Read the model definition and answer for the solid it produces. Units are mm, in the model's axes. Face numbers are marked on the shaded views. Round coordinates to 2 decimals unless told otherwise and drop trailing zeros. Order: outer loops, then holes, each group sorted by start corner. A loop starts at its lowest first (then second) coordinate and runs counter-clockwise, first axis right, second up. Notation, with made-up numbers: (31, 79) -> (52, 79) arc R35 ccw to (52, 113) -> close; hole circle Ø2 at (-39, 24). An arc over 180 degrees is marked (long way). Answer as a JSON object with one key per item and string values. Group by question number.
Item 1: Consider probe 1 along Z at (x, y) = (69, 1.2); probe 2 along X at (y, z) = (1.9, 99); probe 3 along X at (y, z) = (0.6, 98). Determine where each line is inside the solid, lowest interval first. Write a range as from..to.
Item 2: Section A-A, the plane x = -63.5 is taken. Write down the section's boundary in (y, z) (3 decimals), plus the area to 3 significant figures.
Item 3: Given P1, Ø3.5, axis at x = -25.4, z = 189.19, coming from the +Y side, flat-ended and moving along its own axis, determine where the tip first touches the part or whether it passes through.
Item 4: Section B-B, the plane z = 150 is taken. Write down the section's boundary in (x, y) (3 decimals), plus the area to 3 significant figures.
Item 5: Section C-C, the plane y = 1.95 is taken. Count the separate pieces of the cut face and the enclosed holes in it, plus the area to 3 significant figures.
Item 6: Section D-D, the plane x = 91 is taken. Write down the section's boundary in (y, z) (3 decimals), plus the area to 3 significant figures.
Item 7: The mould has two halves that part along Y. Classify the marked faces 1 and 2: pulls with the +Y half, pulls with the -Y half, needs draft (parallel to the pull), parting line crosses it, or undercut.
from build123d import *

# Parameters (mm, degrees)
BOSS_EXTRUDE1_DEPTH = 3.175
CUT_EXTRUDE1_DEPTH  = 252.960239461
BOSS_EXTRUDE2_DEPTH = 3.175
SKETCH4_R           = 2.159
CUT_EXTRUDE2_DEPTH  = 252.960239461


with BuildPart() as part:
    # Sketch1 → Boss-Extrude1 (new body)
    with BuildSketch(Plane(origin=(0, 0, 0), x_dir=(1, 0, 0), z_dir=(0, 1, 0))):
        Polygon((-152.4, 119.059630377), (-116.478975516, 154.980654861), (116.478975516, 154.980654861), (152.4, 119.059630377), (152.4, -164.698320655), (116.478975516, -200.619345139), (-116.478975516, -200.619345139), (-152.4, -164.698320655), align=None)
    extrude(amount=BOSS_EXTRUDE1_DEPTH)

    # Sketch2 → Cut-Extrude1 (cut, through all)
    with BuildSketch(Plane(origin=(0, 3.175, 0), x_dir=(1, 0, 0), z_dir=(0, 1, 0))):
        Polygon((-91.078975516, 129.580654861), (91.078975516, 129.580654861), (127, 93.659630377), (127, 8.930654861), (82.442975516, 8.930654861), (-74.314975516, 8.930654861), (-127, 8.930654861), (-127, 93.659630377), align=None)
        Polygon((127, -139.298320655), (91.078975516, -175.219345139), (-91.078975516, -175.219345139), (-127, -139.298320655), (-127, -54.569345139), (-74.314975516, -54.569345139), (82.442975516, -54.569345139), (127, -54.569345139), align=None)
    extrude(amount=-CUT_EXTRUDE1_DEPTH, mode=Mode.SUBTRACT)

    # Sketch5 → Boss-Extrude2 (add)
    with BuildSketch(Plane(origin=(0, 3.175, 0), x_dir=(1, 0, 0), z_dir=(0, 1, 0))):
        with BuildLine():
            Line((-116.478975516, 83.138605892), (-80.557951031, 119.059630377))
            ThreePointArc((-80.557951031, 119.059630377), (-78.800891411, 126.352814743), (-72.028975516, 129.580654861))
            Line((-72.028975516, 129.580654861), (-59.328975516, 129.580654861))
            Line((-59.328975516, 129.580654861), (-59.328975516, 154.980654861))
            Line((-59.328975516, 154.980654861), (-116.478975516, 154.980654861))
            Line((-116.478975516, 154.980654861), (-152.4, 119.059630377))
            Line((-152.4, 119.059630377), (-152.4, 65.258187686))
            Line((-152.4, 65.258187686), (-127, 65.258187686))
            Line((-127, 65.258187686), (-127, 77.958187686))
            ThreePointArc((-127, 77.958187686), (-123.351279088, 83.821819005), (-116.478975516, 83.138605892))
        make_face()
        with BuildLine():
            Line((127, 65.258187686), (127, 77.958187686))
            ThreePointArc((127, 77.958187686), (123.351279088, 83.821819005), (116.478975516, 83.138605892))
            Line((116.478975516, 83.138605892), (80.557951031, 119.059630377))
            ThreePointArc((80.557951031, 119.059630377), (78.800891411, 126.352814743), (72.028975516, 129.580654861))
            Line((72.028975516, 129.580654861), (59.328975516, 129.580654861))
            Line((59.328975516, 129.580654861), (59.328975516, 154.980654861))
            Line((59.328975516, 154.980654861), (116.478975516, 154.980654861))
            Line((116.478975516, 154.980654861), (152.4, 119.059630377))
            Line((152.4, 119.059630377), (152.4, 65.258187686))
            Line((152.4, 65.258187686), (127, 65.258187686))
        make_face()
        with BuildLine():
            Line((116.478975516, -128.777296171), (80.557951031, -164.698320655))
            ThreePointArc((80.557951031, -164.698320655), (78.800891411, -171.991505021), (72.028975516, -175.219345139))
            Line((72.028975516, -175.219345139), (59.328975516, -175.219345139))
            Line((59.328975516, -175.219345139), (59.328975516, -200.619345139))
            Line((59.328975516, -200.619345139), (116.478975516, -200.619345139))
            Line((116.478975516, -200.619345139), (152.4, -164.698320655))
            Line((152.4, -164.698320655), (152.4, -110.896877964))
            Line((152.4, -110.896877964), (127, -110.896877964))
            Line((127, -110.896877964), (127, -123.596877964))
            ThreePointArc((127, -123.596877964), (123.351279088, -129.460509283), (116.478975516, -128.777296171))
        make_face()
        with BuildLine():
            Line((-127, -110.896877964), (-127, -123.596877964))
            ThreePointArc((-127, -123.596877964), (-123.351279088, -129.460509283), (-116.478975516, -128.777296171))
            Line((-116.478975516, -128.777296171), (-80.557951031, -164.698320655))
            ThreePointArc((-80.557951031, -164.698320655), (-78.800891411, -171.991505021), (-72.028975516, -175.219345139))
            Line((-72.028975516, -175.219345139), (-59.328975516, -175.219345139))
            Line((-59.328975516, -175.219345139), (-59.328975516, -200.619345139))
            Line((-59.328975516, -200.619345139), (-116.478975516, -200.619345139))
            Line((-116.478975516, -200.619345139), (-152.4, -164.698320655))
            Line((-152.4, -164.698320655), (-152.4, -110.896877964))
            Line((-152.4, -110.896877964), (-127, -110.896877964))
        make_face()
    extrude(amount=-BOSS_EXTRUDE2_DEPTH)

    # Sketch4 → Cut-Extrude2 (cut, through all)
    with BuildSketch(Plane(origin=(0, 3.175, 0), x_dir=(1, 0, 0), z_dir=(0, 1, 0))):
        with Locations(Location((0, 143.550654861, 0), (0, 0, 270))):
            Circle(SKETCH4_R)
        with Locations(Location((-50.8, 143.550654861, 0), (0, 0, 270))):
            Circle(SKETCH4_R)
        with Locations(Location((50.8, 143.550654861, 0), (0, 0, 270))):
            Circle(SKETCH4_R)
        with Locations(Location((-25.4, 143.550654861, 0), (0, 0, 270))):
            Circle(SKETCH4_R)
        with Locations(Location((25.4, 143.550654861, 0), (0, 0, 270))):
            Circle(SKETCH4_R)
        with Locations(Location((-140.97, -22.819345139, 0), (0, 0, 270))):
            Circle(SKETCH4_R)
        with Locations(Location((-140.97, 2.580654861, 0), (0, 0, 270))):
            Circle(SKETCH4_R)
        with Locations(Location((-140.97, 27.980654861, 0), (0, 0, 270))):
            Circle(SKETCH4_R)
        with Locations(Location((140.97, -22.819345139, 0), (0, 0, 270))):
            Circle(SKETCH4_R)
        with Locations(Location((140.97, 2.580654861, 0), (0, 0, 270))):
            Circle(SKETCH4_R)
        with Locations(Location((140.97, 27.980654861, 0), (0, 0, 270))):
            Circle(SKETCH4_R)
        with Locations(Location((140.97, -73.619345139, 0), (0, 0, 90))):
            Circle(SKETCH4_R)
        with Locations(Location((140.97, -48.219345139, 0), (0, 0, 90))):
            Circle(SKETCH4_R)
        with Locations(Location((-140.97, -73.619345139, 0), (0, 0, 90))):
            Circle(SKETCH4_R)
        with Locations(Location((-140.97, -48.219345139, 0), (0, 0, 90))):
            Circle(SKETCH4_R)
        with Locations(Location((25.4, -189.189345139, 0), (0, 0, 90))):
            Circle(SKETCH4_R)
        with Locations(Location((-25.4, -189.189345139, 0), (0, 0, 90))):
            Circle(SKETCH4_R)
        with Locations(Location((50.8, -189.189345139, 0), (0, 0, 90))):
            Circle(SKETCH4_R)
        with Locations(Location((-50.8, -189.189345139, 0), (0, 0, 90))):
            Circle(SKETCH4_R)
        with Locations(Location((0, -189.189345139, 0), (0, 0, 90))):
            Circle(SKETCH4_R)
        with Locations(Location((-76.2, 143.550654861, 0), (0, 0, 270))):
            Circle(SKETCH4_R)
        with Locations(Location((76.2, 143.550654861, 0), (0, 0, 270))):
            Circle(SKETCH4_R)
        with Locations(Location((-140.97, 53.380654861, 0), (0, 0, 270))):
            Circle(SKETCH4_R)
        with Locations(Location((140.97, 53.380654861, 0), (0, 0, 270))):
            Circle(SKETCH4_R)
        with Locations(Location((140.97, -99.019345139, 0), (0, 0, 90))):
            Circle(SKETCH4_R)
        with Locations(Location((76.2, -189.189345139, 0), (0, 0, 90))):
            Circle(SKETCH4_R)
        with Locations(Location((-76.2, -189.189345139, 0), (0, 0, 90))):
            Circle(SKETCH4_R)
        with Locations(Location((-140.97, -99.019345139, 0), (0, 0, 90))):
            Circle(SKETCH4_R)
    extrude(amount=-CUT_EXTRUDE2_DEPTH, mode=Mode.SUBTRACT)


solid = part.part
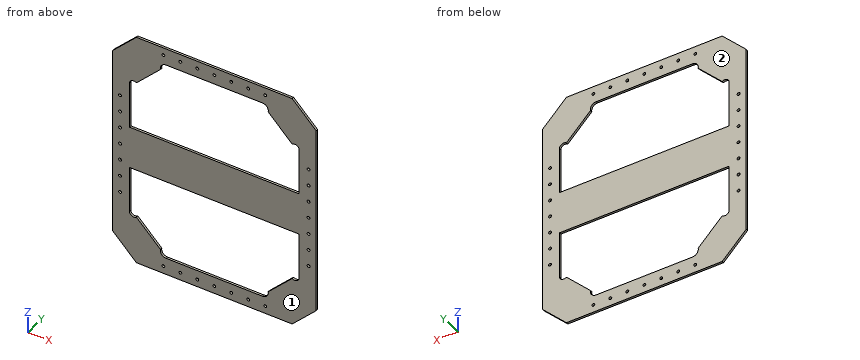
Values found:
{
 "1": {"probe 1": "-154.98..-129.58, -8.93..54.57, 175.22..200.62", "probe 2": "-152.4..-143.13, -138.81..-127, 127..138.81, 143.13..152.4", "probe 3": "-152.4..-142.87, -139.07..-127, 127..139.07, 142.87..152.4"},
 "2": {"outline": "(0, -154.981) -> (3.175, -154.981) -> (3.175, -129.581) -> (0, -129.581) -> close; (0, -8.931) -> (3.175, -8.931) -> (3.175, 54.569) -> (0, 54.569) -> close; (0, 175.219) -> (3.175, 175.219) -> (3.175, 200.619) -> (0, 200.619) -> close", "area": "363 mm2"},
 "3": {"P1": "through"},
 "4": {"outline": "(-152.4, 0) -> (-95.256, 0) -> (-95.256, 3.175) -> (-152.4, 3.175) -> close; (95.256, 0) -> (152.4, 0) -> (152.4, 3.175) -> (95.256, 3.175) -> close", "area": "363 mm2"},
 "5": {"separate pieces": "1", "enclosed holes": "30", "area": "50,200 mm2"},
 "6": {"outline": "(0, -154.981) -> (3.175, -154.981) -> (3.175, -108.618) -> (0, -108.618) -> close; (0, -8.931) -> (3.175, -8.931) -> (3.175, 54.569) -> (0, 54.569) -> close; (0, 154.256) -> (3.175, 154.256) -> (3.175, 200.619) -> (0, 200.619) -> close", "area": "496 mm2"},
 "7": {"face 1": "pulls with the -Y half", "face 2": "pulls with the +Y half"}
}
